```python
from build123d import *

# Parameters (mm, degrees)
F0_R     = 5
F1_DEPTH = 9.5


with BuildPart() as f1:
    # F0 (on Top) → F1 (new body)
    with BuildSketch(Plane.XY):
        with BuildLine():
            ThreePointArc((251.4837984218, 174.4078397694), (245.9373500957, 178.9093807212), (238.8024981834, 178.5617484971))
            Line((238.8024981834, 178.5617484971), (139.4635551595, 134.9226100063))
            Line((139.4635551595, 134.9226100063), (127.3100964327, 129.5836517652))
            ThreePointArc((127.3100964327, 129.5836517652), (116.6299314638, 128.0692059728), (106.7166346632, 132.3219717036))
            ThreePointArc((106.7166346632, 132.3219717036), (82.8740793121, 148.410763694), (56.6604115001, 160.2496949469))
            ThreePointArc((56.6604115001, 160.2496949469), (47.6215255634, 166.7206128225), (43.4338375319, 177.0180642585))
            Line((43.4338375319, 177.0180642585), (30.2674388345, 302.399259814))
            ThreePointArc((30.2674388345, 302.399259814), (27.1466203514, 304.3271806603), (23.5405558858, 305))
            Line((23.5405558858, 305), (-0.0569906184, 305))
            Line((-0.0569906184, 305), (-0.0663333427, 305))
            Line((-0.0663333427, 305), (-0.0663333427, 355))
            Line((-0.0663333427, 355), (-50.0663333427, 355))
            Line((-50.0663333427, 355), (-50.0663333427, 127.0140681159))
            Line((-50.0663333427, 127.0140681159), (134.9963067562, 20.2325334796))
            Line((134.9963067562, 20.2325334796), (332.3060807422, 134.1985475298))
            Line((332.3060807422, 134.1985475298), (307.2979901421, 177.495145601))
            Line((307.2979901421, 177.495145601), (264.1092482344, 152.5493526602))
            Line((264.1092482344, 152.5493526602), (251.4837984218, 174.4078397694))
        make_face()
        with BuildLine():
            ThreePointArc((59.8321268024, 103.7222201288), (59.8304304841, 112.3828004264), (67.3309958809, 108.0529998887))
            ThreePointArc((67.3309958809, 108.0529998887), (64.8315612777, 103.723199351), (59.8321268024, 103.7222201288))
        make_face(mode=Mode.SUBTRACT)
        with Locations((276.5054373709, 130.8387559654)):
            Circle(F0_R, mode=Mode.SUBTRACT)
        with Locations((-25.0663333427, 305)):
            Circle(F0_R, mode=Mode.SUBTRACT)
        Polygon((-0.0663333427, 305), (-0.0569906184, 305), (-0.0663333427, 355), align=None)
    extrude(amount=F1_DEPTH)


solid = f1.part
```
Input: part model. Units: mm. Frame: model coordinates. A direction names the side the tool comes from. Coordinates: 2 decimals unless noted, no trailing zeros. Loops run counter-clockwise (first coordinate to the right, second up) from the corner with the lowest first, then second, coordinate; pieces in that order, holes last. Notation, with made-up numbers: M 88.25,84 L 115.25,84 A20 ccw 115.25,114 Z; hole C -25.5,82 d2. An arc over 180 degrees is marked long. Answer in a Markdown table with one row per item.
1. Material intervals for line 1 (X direction, y = 135, z = 7.75); line 2 (X direction, y = 331.5, z = 3.5); line 3 (X direction, y = 308.5, z = 8.75), sorted ascending.
Response:
| item | result |
|---|---|
| line 1 | x = -50.07 to 103.31, 139.64 to 273.73, 279.28 to 331.84 |
| line 2 | x = -50.07 to -0.06 |
| line 3 | x = -50.07 to -28.64, -21.5 to -0.06 |
2. Section A-A, the plane z = 8. Output: boundary loops of the cut face in (x, y), then the cut area to 3 significant figures.
Response:
| item | result |
|---|---|
| outline | M -50.07,127.01 L 135,20.23 L 332.31,134.2 L 307.3,177.5 L 264.11,152.55 L 251.48,174.41 A10 ccw 238.8,178.56 L 127.31,129.58 A20 cw 106.72,132.32 A170 ccw 56.66,160.25 A20 cw 43.43,177.02 L 30.27,302.4 A10 ccw 23.54,305 L -0.06,305 L -0.07,355 L -50.07,355 Z; hole C -25.07,305 d10; hole C 62.33,108.05 d10; hole C 276.51,130.84 d10 |
| area | 45,800 mm2 |
3. Draft query along Y for faces 4 (the flat face through (183.8, 154.4, 4.7)), 5 (the cylindrical face through (-25.717, 309.957, 4.684)), 6 (the flat face through (97.7, 138.8, 9.5)), 7 (the cylindrical face through (271.51, 131.06, 4.68)). Return one class per face: pulls with the +Y half, pulls with the -Y half, needs draft (parallel to the pull), parting line crosses it, or undercut.
Response:
| item | result |
|---|---|
| face 4 | pulls with the +Y half |
| face 5 | undercut |
| face 6 | needs draft |
| face 7 | undercut |
4. Section C-C, the plane x = 141.5. Output: boundary loops of the cut face in (y, z).
Response:
| item | result |
|---|---|
| outline | M 23.99,0 L 135.82,0 L 135.82,9.5 L 23.99,9.5 Z |
5. Section B-B, the plane y = 253. Output: boundary loops of the cut face in (x, z), then the cut area to 3 significant figures.
Response:
| item | result |
|---|---|
| outline | M -50.07,0 L 35.45,0 L 35.45,9.5 L -50.07,9.5 Z |
| area | 812 mm2 |
6. Reachability of faces 1 (the flat face through (12, 305, 5)), 2 (the flat face through (232.27, 76.42, 4.68)), 3 (the cylindrical face through (47.72, 166.597, 4.684)) from +Z, -Z, +X, -X, +Y, -Y: full face, straight path, thin tool, end or side. Return the list, or none.
Response:
| item | result |
|---|---|
| face 1 | +Z, -Z, +X, +Y |
| face 2 | +Z, -Z, +X, -Y |
| face 3 | +Z, -Z, +Y |
7. First-contact query: pin 1 (2 mm diameter, centred on x = 142, y = 128.5, fed in from -Z); pin 2 (2 mm diameter, centred on y = 76, z = 3.5, fed in from -X); pin 3 (3 mm diameter, centred on x = 13, z = 4.5, fed in from +Y); pin 4 (3 mm diameter, centred on x = 86, z = 3, fed in from -Y). Flat tips, straight axial feed; report the tip coordinate or a pass-through.
Response:
| item | result |
|---|---|
| pin 1 | stops at z = 0 |
| pin 2 | stops at x = 36.61 |
| pin 3 | stops at y = 305 |
| pin 4 | stops at y = 47.64 |
